from build123d import *

# Parameters (mm, degrees)
F1_DEPTH = 25.4
F2_DEPTH = 12.7
F4_DEPTH = 25.4
F6_DEPTH = 25.4


with BuildPart() as f1:
    # F0 (on Top) → F1 (new body)
    with BuildSketch(Plane.XY):
        Polygon((38.1, 25.4), (25.4, 25.4), (25.4, 12.7), (25.4, 0), (38.1, 0), align=None)
    extrude(amount=F1_DEPTH)

    # F0 (on Top) → F2 (join)
    with BuildSketch(Plane.XY):
        Polygon((0, 25.4), (0, 0), (12.7, 0), (12.7, 12.7), (25.4, 12.7), (25.4, 25.4), align=None)
        Polygon((38.1, 25.4), (25.4, 25.4), (25.4, 12.7), (25.4, 0), (38.1, 0), align=None)
    extrude(amount=F2_DEPTH)

    # F3 (on face) → F4 (cut)
    with BuildSketch(Plane.YZ.offset(12.7)):
        Polygon((0, 0), (6.35, 12.7), (0, 12.7), align=None)
    extrude(amount=-F4_DEPTH, mode=Mode.SUBTRACT)

    # F5 (on face) → F6 (cut)
    with BuildSketch(Plane.YZ.offset(38.1)):
        Polygon((0, 12.7), (12.7, 25.4), (0, 25.4), align=None)
    extrude(amount=-F6_DEPTH, mode=Mode.SUBTRACT)


solid = f1.part
Design review of the part built by this model. Coordinates are the model's own, in mm. A direction names the side the tool comes from. Coordinates: 2 decimals unless noted, no trailing zeros. Loops run counter-clockwise (first coordinate to the right, second up) from the corner with the lowest first, then second, coordinate; pieces in that order, holes last.
Item 1: Add section A-A (y = 8.5). Write out the cut boundary in (x, z).
Completed:
outline: (0, 0) - (12.7, 0) - (12.7, 12.7) - (0, 12.7) - close; (25.4, 0) - (38.1, 0) - (38.1, 21.2) - (25.4, 21.2) - close
Item 2: Add section C-C (x = 29). Write out the cut boundary in (y, z).
Completed:
outline: (0, 0) - (25.4, 0) - (25.4, 25.4) - (12.7, 25.4) - (0, 12.7) - close
Item 3: Wall thickness on L1, parallel to X at y = 8.5, z = 12.25; L2, parallel to Z at x = 18, y = 17; L3, parallel to X at y = 5.5, z = 15.75: over which ranges is each line inside the solid? List them lowest first.
Completed:
L1: x = 0 to 12.7, 25.4 to 38.1
L2: z = 0 to 12.7
L3: x = 25.4 to 38.1
Item 4: Clearance check with flat-ended pins moving along their axes: pin 1 (12 mm diameter, centred on y = 13.5, z = 20, fed in from -X); pin 2 (4 mm diameter, centred on x = 17, z = 9, fed in from -Y); pin 3 (6 mm diameter, centred on x = 13, y = 8, fed in from +Z). State where each tip first meets the part, or that it passes through.
Completed:
pin 1: stops at x = 25.4
pin 2: stops at y = 12.7
pin 3: stops at z = 12.7
Item 5: Add section B-B (y = 2). Write out the cut boundary in (x, z), and give its area (3 significant figures).
Completed:
outline: (0, 0) - (12.7, 0) - (12.7, 4) - (0, 4) - close; (25.4, 0) - (38.1, 0) - (38.1, 14.7) - (25.4, 14.7) - close
area: 237 mm2
Item 6: For faces 1 (the flat face through (12.7, 8, 6)), 2 (the flat face through (25.4, 10, 13)), 3 (the flat face through (0, 16, 6)), 4 (the flat face through (13, 18, 12.7)), list the 3-axis set-ups (+Z, -Z, +X, -X, +Y, -Y) from which the entire face can be reached by the end or side of a thin tool; tool diameter is ignored.
Completed:
face 1: +Z, -Z, -Y
face 2: +Z, -Y
face 3: +Z, -Z, -X, +Y, -Y
face 4: +Z, -X, +Y, -Y
Item 7: Add section D-D (z = 16.75). Write out the cut boundary in (x, y), and give its area (3 significant figures).
Completed:
outline: (25.4, 4.05) - (38.1, 4.05) - (38.1, 25.4) - (25.4, 25.4) - close
area: 271 mm2
Item 8: Draft analysis for pull direction X (two halves, no side actions). For faces 5 (the flat face through (6, 3, 6)), 6 (the flat face through (38.1, 13, 13)), 7 (the flat face through (19, 12.7, 6)), state which applies: pulls with the +X half, pulls with the -X half, needs draft (parallel to the pull), parting line crosses it, or undercut.
Completed:
face 5: needs draft
face 6: pulls with the +X half
face 7: undercut
